Could you check a few things on this model? Use its own coordinates, in mm. A direction names the side the tool comes from. Coordinates: 2 decimals unless noted, no trailing zeros. Loops run counter-clockwise (first coordinate to the right, second up) from the corner with the lowest first, then second, coordinate; pieces in that order, holes last.
from build123d import *

# Parameters (mm, degrees)
F1_DEPTH = 2


# Not quite as in the source:
# - a feature names something its author has since deleted; it is built from what else it names


with BuildPart() as f1:
    # F0 (on Top) → F1 (new body)
    with BuildSketch(Plane.XY):
        Polygon((63.5912331811, -12.2381385313), (63.3644544975, -11.5834848612), (43.3012701892, 0), (43.3012701892, 46.333939444), (42.3941554539, 48.9525541272), (41.7138194028, 49.0834848613), (21.6506350946, 37.5000000002), (-18.4757335211, 60.6669697221), (-21.1970777272, 61.1906926587), (-21.6506350946, 60.6669697224), (-21.6506350946, 37.5), (-61.7770037106, 14.333030278), (-63.591233181, 12.2381385317), (-63.3644544972, 11.583484861), (-43.3012701894, 1e-10), (-43.3012701894, -46.3339394428), (-42.3941554538, -48.9525541268), (-41.7138194016, -49.0834848611), (-21.6506350939, -37.5000000002), (18.4757335209, -60.6669697216), (21.1970777272, -61.1906926583), (21.6506350946, -60.666969722), (21.6506350946, -37.5), (61.7770037099, -14.3330302784), align=None)
        Polygon((19.6506350946, -36.3452994616), (19.6506350946, -59.0358983857), (-19.6506350948, -36.3452994623), (5e-10, -25.0000000003), align=None, mode=Mode.SUBTRACT)
        Polygon((-1.0000000004, 0.5773502687), (-1.9999999999, -2e-10), (-22.6506350946, -11.9226497308), (-1.9999999997, -23.8452994618), (-41.3012701889, -46.535898385), (-41.3012701889, -1.1547005386), (-1.0000000004, 22.1132486534), (-1.0000000004, 1.7320508071), align=None, mode=Mode.SUBTRACT)
        Polygon((21.6506350946, 10.1905989232), (60.9519052838, -12.5), (21.6506350946, -35.1905989232), (-18.6506350946, -11.9226497308), (-1, -1.7320508076), (0, -1.1547005384), (21.6506350946, -13.6547005384), align=None, mode=Mode.SUBTRACT)
        Polygon((-60.9519052838, 12.5), (-21.6506350946, 35.1905989232), (-21.6506350946, 12.5000000002), (-41.3012701894, 1.1547005385), align=None, mode=Mode.SUBTRACT)
        Polygon((19.6506350946, -10.1905989242), (2, -1e-09), (1.0000000005, 0.5773502699), (1.0000000005, 1.7320508081), (1.0000000005, 25.5773502697), (-19.6506350952, 13.6547005382), (-19.6506350952, 59.0358983854), (19.6506350946, 36.3452994618), align=None, mode=Mode.SUBTRACT)
        Polygon((21.6506350946, 35.1905989229), (41.3012701896, 46.5358983847), (41.3012701896, 1.1547005382), (21.6506350946, 12.5), align=None, mode=Mode.SUBTRACT)
        Polygon((-21.6506350946, 60.6669697224), (-21.6506350946, 62.5000000002), (-64.9519052838, 12.5), (-61.7770037106, 14.333030278), align=None)
        Polygon((41.7138194028, 49.0834848613), (43.3012701892, 50.0000000002), (-21.6506350948, 62.5000000001), (-18.4757335211, 60.6669697221), align=None)
        Polygon((-64.9519052838, 12.5), (-43.301270189, -50), (-43.3012701894, -46.3339394428), (-63.3644544972, 11.583484861), align=None)
        Polygon((-61.7770037106, 14.333030278), (-64.9519052838, 12.5), (-63.3644544972, 11.583484861), (-63.591233181, 12.2381385317), align=None)
        Polygon((-43.3012701894, -46.3339394428), (-43.3012701894, -50.0000000007), (-41.7138194016, -49.0834848611), (-42.3941554538, -48.9525541268), align=None)
        Polygon((-43.301270189, -50), (21.6506350949, -62.4999999997), (18.4757335209, -60.6669697216), (-41.7138194016, -49.0834848611), align=None)
        Polygon((18.4757335209, -60.6669697216), (21.6506350946, -62.4999999998), (21.6506350946, -60.666969722), (21.1970777272, -61.1906926583), align=None)
        Polygon((21.6506350949, -62.4999999997), (64.9519052839, -12.4999999995), (61.7770037099, -14.3330302784), (21.6506350946, -60.666969722), align=None)
        Polygon((61.7770037099, -14.3330302784), (64.9519052838, -12.5), (63.3644544975, -11.5834848612), (63.5912331811, -12.2381385313), align=None)
        Polygon((63.3644544975, -11.5834848612), (64.9519052838, -12.5), (43.3012701891, 50.0000000004), (43.3012701892, 46.333939444), align=None)
        Polygon((43.3012701892, 46.333939444), (43.3012701892, 50.0000000002), (41.7138194028, 49.0834848613), (42.3941554539, 48.9525541272), align=None)
        Polygon((-18.4757335211, 60.6669697221), (-21.6506350946, 62.5000000002), (-21.6506350946, 60.6669697224), (-21.1970777272, 61.1906926587), align=None)
    extrude(amount=F1_DEPTH)


solid = f1.part
(1) Imagine slicing it at B-B, the plane x = 13.5. Write out the boundary of the cut face in (y, z), and give its area (3 significant figures).
Answers:
outline: (-60.93, 0) - (-59.71, 0) - (-59.71, 2) - (-60.93, 2) - close; (-57.79, 0) - (-55.48, 0) - (-55.48, 2) - (-57.79, 2) - close; (-32.79, 0) - (-30.48, 0) - (-30.48, 2) - (-32.79, 2) - close; (-8.95, 0) - (-6.64, 0) - (-6.64, 2) - (-8.95, 2) - close; (39.9, 0) - (42.21, 0) - (42.21, 2) - (39.9, 2) - close; (54.51, 0) - (55.74, 0) - (55.74, 2) - (54.51, 2) - close
area: 23.4 mm2
(2) We'd pull the mould along X, two halves only. Please class faces 3 (the face through (0, 0, 2)), 4 (the face through (-54.28, -18.31, 0.99)), 5 (the face through (-0.28, 47.85, 0.99)): +X half, -X half, draft (parallel to the pull), parting line (faces both ways), or undercut.
Answers:
face 3: draft
face 4: -X half
face 5: undercut
(3) Imagine slicing it at A-A, the plane x = 34. Write out the boundary of the cut face in (y, z).
Answers:
outline: (-48.24, 0) - (-46.41, 0) - (-46.41, 2) - (-48.24, 2) - close; (-30.37, 0) - (-28.06, 0) - (-28.06, 2) - (-30.37, 2) - close; (3.06, 0) - (5.37, 0) - (5.37, 2) - (3.06, 2) - close; (42.32, 0) - (44.63, 0) - (44.63, 2) - (42.32, 2) - close; (50.57, 0) - (51.79, 0) - (51.79, 2) - (50.57, 2) - close
(4) Which directions (+Z, -Z, +X, -X, +Y, -Y) give clear straight access to the entire face, cutting with the end or side of a thin tool? Please do faces 1 (the face through (11.28, 56.163, 0.986)), 2 (the face through (-9.96, -30.75, 0.99)).
Answers:
face 1: +Z, -Z, +X, +Y
face 2: +Z, -Z
(5) I need wall thicknesses on probe 1 along Y at (x, z) = (-29, 1.8); probe 2 along X at (y, z) = (28, 0.75); probe 3 along X at (y, z) = (26, 0.9). Which ranges of each line are inside material? Lowest first, please.
Answers:
probe 1: y = -52.75 to -51.53, -41.74 to -39.43, 5.95 to 8.26, 30.95 to 33.26, 52.18 to 54.01
probe 2: x = -51.53 to -49.94, -38.11 to -34.11, -21.65 to -19.65, 19.65 to 21.65, 41.3 to 43.3, 49.65 to 50.92
probe 3: x = -53.26 to -51.67, -41.57 to -37.57, -21.65 to -19.65, 19.65 to 21.65, 41.3 to 43.3, 50.35 to 51.62
(6) Imagine slicing it at C-C, the plane z = 1.25. State how many separate pieces and enclosed holes the cut face has, and give its area (3 significant figures).
Answers:
separate pieces: 1
enclosed holes: 12
area: 1,890 mm2
(7) For pin 1 (0.6 mm diameter, centred on y = 28.5, z = 0.5, fed in from -X); pin 2 (0.6 mm diameter, centred on y = -2.5, z = 0.5, fed in from +X); pin 3 (0.6 mm diameter, centred on y = 21, z = 0.5, fed in from +X); pin 4 (12 mm diameter, centred on x = 39.5, y = -36, fed in from -Z), each with a flat end and sliding along its axis, tell me the tip position at first contact or that it passes through.
Answers:
pin 1: stops at x = -51.36
pin 2: stops at x = 61.59
pin 3: stops at x = 53.45
pin 4: stops at z = 0
